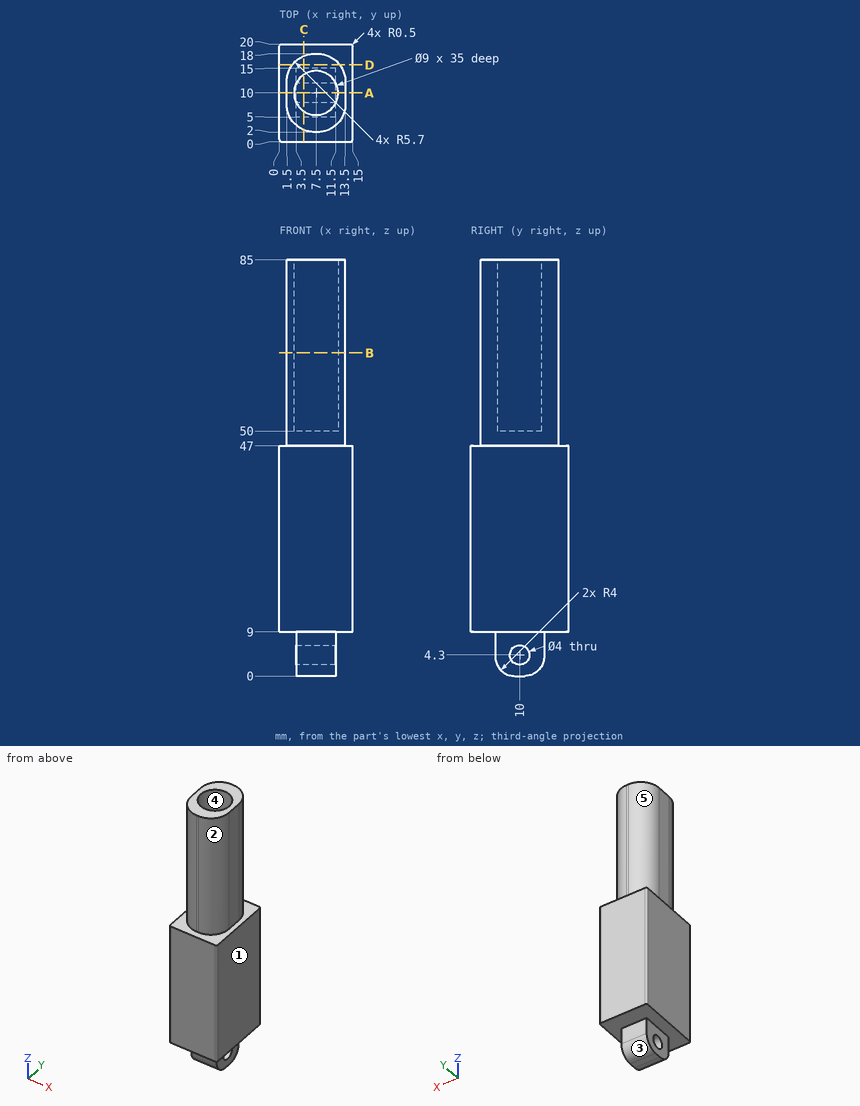
Here's the drawing with two shaded views (mm, measured from the low corner). I have some questions. A direction names the side the tool comes from. Give positions to 0.01 mm unless a question says otherwise; leave off trailing zeros. Order: outer loops, then holes, each group sorted by start corner. A loop starts at its lowest first (then second) coordinate and runs counter-clockwise, first axis right, second up. Notation, with made-up numbers: (8, 72) - (42, 72) arc R27 cw to (42, 107) - close; hole circle Ø6 at (64, 23). An arc over 180 degrees is marked (long way). Use a Markdown table: item, result. Add a question column.
Q1. If we section it at B-B on z = 66: Write out the boundary of the cut face in (x, y).
Q2. If we section it at A-A on y = 10: Write out the boundary of the cut face in (x, z), plus the area to 3 significant figures.
Q3. If we section it at C-C on x = 5: Write out the boundary of the cut face in (y, z).
Q4. I'm going to push flat-ended pins straight in: pin 1 (4.5 mm diameter, centred on y = 9, z = 4.5, fed in from -X); pin 2 (5 mm diameter, centred on x = 3, z = 56, fed in from -Y); pin 3 (6.5 mm diameter, centred on y = 10, z = 4.3, fed in from +X). Where does each tip first touch, or does it pass through?
Q5. If we mould it in two halves opening along X, with no side actions, what happens to the marked faces 3, 4 and 5? For each: released by +X, released by -X, zero draft, split by the parting line, or undercut.
Q6. On a 3-axis mill with a long thin cutter (end or side, diameter ignored), from which of +Z, -Z, +X, -X, +Y, -Y can I reach the whole of each face in a straight line? I mean the marked faces 1 and 2. Say none if no direction works.
Q7. Please list where these lines run through material, in increasing order: line 1 along Y through (x, z) = (7, 4.3); line 2 along Y through (x, z) = (7.5, 72.5); line 3 along Z through (x, y) = (9.75, 9.25).
Q8. If we section it at D-D on y = 15.75: Write out the boundary of the cut face in (x, z).
Answers follow:
| question | item | result |
|---|---|---|
| 1 | outline | (1.5, 7.7) arc R5.7 ccw to (7.2, 2) - (7.8, 2) arc R5.7 ccw to (13.5, 7.7) - (13.5, 12.3) arc R5.7 ccw to (7.8, 18) - (7.2, 18) arc R5.7 ccw to (1.5, 12.3) - close; hole circle Ø9 at (7.5, 10) |
| 2 | outline | (0, 9) - (3.5, 9) - (3.5, 6.3) - (11.5, 6.3) - (11.5, 9) - (15, 9) - (15, 47) - (13.5, 47) - (13.5, 85) - (12, 85) - (12, 50) - (3, 50) - (3, 85) - (1.5, 85) - (1.5, 47) - (0, 47) - close; (3.5, 0) - (11.5, 0) - (11.5, 2.3) - (3.5, 2.3) - close |
| 2 | area | 751 mm^2 |
| 3 | outline | (0, 9) - (5, 9) - (5, 4) arc R4 ccw to (9, 0) - (11, 0) arc R4 ccw to (15, 4) - (15, 9) - (20, 9) - (20, 47) - (17.56, 47) - (17.56, 85) - (13.74, 85) - (13.74, 50) - (6.26, 50) - (6.26, 85) - (2.44, 85) - (2.44, 47) - (0, 47) - close; hole circle Ø4 at (10, 4.3) |
| 4 | pin 1 | stops at x = 3.5 |
| 4 | pin 2 | stops at y = 2.26 |
| 4 | pin 3 | stops at x = 11.5 |
| 5 | face 3 | zero draft |
| 5 | face 4 | undercut |
| 5 | face 5 | released by -X |
| 6 | face 1 | +Z, -Z, +X, +Y, -Y |
| 6 | face 2 | +Z, +X, -Y |
| 7 | line 1 | y = 5 to 8, 12 to 15 |
| 7 | line 2 | y = 2 to 5.5, 14.5 to 18 |
| 7 | line 3 | z = 0 to 2.45, 6.15 to 50 |
| 8 | outline | (0, 9) - (15, 9) - (15, 47) - (12.34, 47) - (12.34, 85) - (2.66, 85) - (2.66, 47) - (0, 47) - close |
